Could you check a few things on this model? Use its own coordinates, in mm. Give positions to 0.01 mm unless a question says otherwise; leave off trailing zeros. Write each loop counter-clockwise with the first axis right and the second up, starting at its lowest first coordinate (ties: lowest second). Pieces come first, ordered by that corner, then holes. Notation, with made-up numbers: M 24.5,80.25 L 52.5,80.25 A15 cw 52.5,99.25 Z; hole C 10,1.25 d2. An arc over 180 degrees is marked long. One line per item, written item: value.
Autodesk Inventor part; units mm, degrees
ref_plane "YZ Plane" through (0, 0, 0) normal (1, 0, 0) x (0, 1, 0)
ref_plane "XZ Plane" through (0, 0, 0) normal (0, 1, 0) x (-1, 0, 0)
ref_plane "XY Plane" through (0, 0, 0) normal (0, 0, 1) x (1, 0, 0)
sketch "Sketch1" plane through (0, 0, 0) normal (0, 1, 0) x (-1, 0, 0)
  circle A0 centre (0, 0) radius 30
  circle A1 centre (0, 0) radius 12.7
  dimension "d1" = 60
  dimension "d14" = 25.4
extrude "Extrusion1" add sketch "Sketch1" along normal blind 20 contours A0 | A1
extrude "Extrusion2" cut sketch "Sketch1" along normal blind 11.4 contours A1
chamfer "Chamfer2" distance 11.4 distance2 7.5 1 edges at (12.7, 11.4, 0) measured on face at (-12.5355, 7.6, -2.0372)
sketch "Sketch2" plane through (0, 11.4, 0) normal (0, -1, 0) x (1, 0, 0)
  circle A0 centre (0, 0) radius 5.2
extrude "Extrusion3" cut sketch "Sketch2" against normal blind 11.4
properties part number "1. ring"
1) If we section it at D-D, the plane y = 7.75: Write out the boundary of the cut face in (x, z), then the cut area to 3 significant figures.
Outcome:
outline: C 0,0 d60; hole C 0,0 d15.2
area: 2,650 mm^2
2) If we section it at C-C, the plane y = 17.25: Write out the boundary of the cut face in (x, z), then the cut area to 3 significant figures.
Outcome:
outline: C 0,0 d60; hole C 0,0 d10.4
area: 2,740 mm^2
3) Please list where these lines run through material, in increasing order: L1, parallel to Z at x = 0, y = 17.75; L2, parallel to X at y = 11, z = 2; L3, parallel to Z at x = 10.5, y = 1.5. Write a range as from..to.
Outcome:
L1: z = -30..-5.2, 5.2..30
L2: x = -29.93..-5.08, 5.08..29.93
L3: z = -28.1..-5.19, 5.19..28.1
4) We'd pull the mould along Z, two halves only. Please class faces 1 (the face through (0, 0, -13)), 2 (the face through (29.97, 9.86, -1.32)), 3 (the face through (-0.677, 15.64, 5.156)): pulls with the +Z half, pulls with the -Z half, needs draft (parallel to the pull), parting line crosses it, or undercut.
Outcome:
face 1: needs draft
face 2: parting line crosses it
face 3: undercut
5) I'm going to push flat-ended pins straight in: pin 1 (2 mm diameter, centred on x = -11, y = 7, fed in from +Z); pin 2 (1 mm diameter, centred on y = 8.5, z = -6.5, fed in from +X); pin 3 (12 mm diameter, centred on y = 5, z = 10.5, fed in from -X). Where does each tip first touch, or does it pass through?
Outcome:
pin 1: stops at z = 28.28
pin 2: stops at x = 29.39
pin 3: stops at x = -29.66
